CAD build for the part. Positions are in the model's coordinates, mm. Give positions to 0.01 mm unless a question says otherwise; leave off trailing zeros. Write each loop counter-clockwise with the first axis right and the second up, starting at its lowest first coordinate (ties: lowest second). Pieces come first, ordered by that corner, then holes. Notation, with made-up numbers: (31, 32.5) - (47, 32.5) arc R13 ccw to (47, 56.5) - close; hole circle Ø11 at (20, 53). An arc over 180 degrees is marked (long way). Write item = value, one per line. Start each with the question number.
```python
from build123d import *

# Parameters (mm, degrees)
Y_KSEKLIK_EKSTR_ZYON1_DEPTH = 100
IZIM6_R                     = 3
KES_EKSTR_ZYON2_DEPTH       = 1
KES_EKSTR_ZYON2_DEPTH_BACK  = 101


with BuildPart() as part:
    # Çizim4 → Yükseklik-Ekstrüzyon1 (new body)
    with BuildSketch(Plane.XY):
        with BuildLine():
            Line((-3.666174594, 6.349999778), (-1.581220903, 6.349999778))
            ThreePointArc((-1.581220903, 6.349999778), (-3.85e-07, 4.768779481), (1.581220134, 6.349999778))
            Line((1.581220134, 6.349999778), (3.666173825, 6.349999778))
            Line((3.666173825, 6.349999778), (4.708650587, 4.544377312))
            ThreePointArc((4.708650587, 4.544377312), (4.129884032, 2.384389991), (6.289871272, 1.805623132))
            Line((6.289871272, 1.805623132), (7.332348419, 0))
            Line((7.332348419, 0), (6.289871875, -1.805622592))
            ThreePointArc((6.289871875, -1.805622592), (4.12988432, -2.384389491), (4.708651522, -4.544376964))
            Line((4.708651522, -4.544376964), (3.666174594, -6.350000222))
            Line((3.666174594, -6.350000222), (1.581220903, -6.350000222))
            ThreePointArc((1.581220903, -6.350000222), (3.85e-07, -4.768779481), (-1.581220134, -6.350000222))
            Line((-1.581220134, -6.350000222), (-3.666173825, -6.350000222))
            Line((-3.666173825, -6.350000222), (-4.708650779, -4.544377423))
            ThreePointArc((-4.708650779, -4.544377423), (-4.129884032, -2.384389991), (-6.289871464, -1.805623243))
            Line((-6.289871464, -1.805623243), (-7.332348419, -4.44e-07))
            Line((-7.332348419, -4.44e-07), (-6.289871683, 1.805622481))
            ThreePointArc((-6.289871683, 1.805622481), (-4.12988432, 2.384389491), (-4.70865133, 4.544376853))
            Line((-4.70865133, 4.544376853), (-3.666174594, 6.349999778))
        make_face()
    extrude(amount=Y_KSEKLIK_EKSTR_ZYON1_DEPTH)

    # Çizim6 → Kes-Ekstrüzyon2 (cut, two sides)
    with BuildSketch(Plane(origin=(0, 0, 0), x_dir=(-1, 0, 0), z_dir=(0, 0, -1))) as kes_ekstr_zyon2_sk:
        Circle(IZIM6_R)
    extrude(amount=KES_EKSTR_ZYON2_DEPTH, mode=Mode.SUBTRACT)
    extrude(kes_ekstr_zyon2_sk.sketch, amount=-KES_EKSTR_ZYON2_DEPTH_BACK, mode=Mode.SUBTRACT)


solid = part.part
```
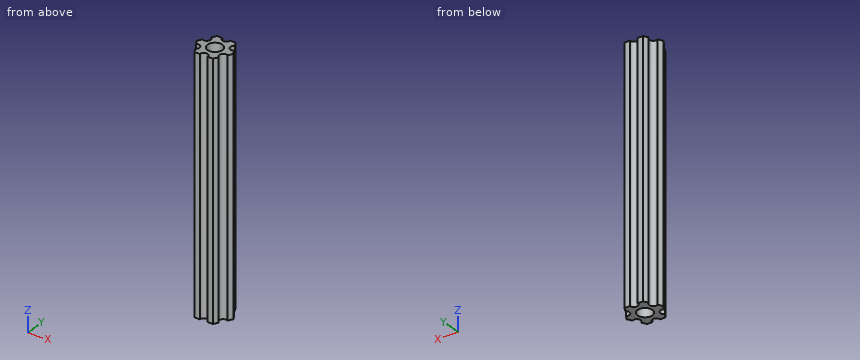
1. Cut at A-A (z = 80). Give the cut face in (x, y) (3 decimals).
2. Cut at B-B (x = 0). Give the cut face in (y, z), then the cut area to 3 significant figures.
3. Wall check: line 1 along Y through (x, z) = (0, 35); line 2 along Y through (x, z) = (4.5, 82); line 3 along Y through (x, z) = (-2.25, 21). Give the ranges that are in metal, low to high.
4. Pin check, flat tip, straight feed: pin 1 Ø4 at (y, z) = (-3, 78.5) entering from +X (3 decimals). Stop position of the tip, or through.
Output:
q1.outline = (-7.332, 0) - (-6.29, -1.806) arc R1.581 cw to (-4.709, -4.544) - (-3.666, -6.35) - (-1.581, -6.35) arc R1.581 cw to (1.581, -6.35) - (3.666, -6.35) - (4.709, -4.544) arc R1.581 cw to (6.29, -1.806) - (7.332, 0) - (6.29, 1.806) arc R1.581 cw to (4.709, 4.544) - (3.666, 6.35) - (1.581, 6.35) arc R1.581 cw to (-1.581, 6.35) - (-3.666, 6.35) - (-4.709, 4.544) arc R1.581 cw to (-6.29, 1.806) - close; hole circle Ø6 at (0, 0)
q2.outline = (-4.77, 0) - (-3, 0) - (-3, 100) - (-4.77, 100) - close; (3, 0) - (4.77, 0) - (4.77, 100) - (3, 100) - close
q2.area = 354 mm2
q3.line_1 = -4.77 to -3, 3 to 4.77
q3.line_2 = -4.91 to -4.4, -1.95 to 1.95, 4.4 to 4.91
q3.line_3 = -6.35 to -1.98, 1.98 to 6.35
q4.pin_1 = 6.755
